For this review, use the dimensioned drawing (mm, ordinates from the lowest corner) and the shaded views. Coordinates: 2 decimals unless noted, no trailing zeros. Loops run counter-clockwise (first coordinate to the right, second up) from the corner with the lowest first, then second, coordinate; pieces in that order, holes last. Notation, with made-up numbers: (0, 32) - (45, 32) arc R18 cw to (45, 37) - close; hole circle Ø10 at (-1.5, -34). An arc over 180 degrees is marked (long way). Answer in a Markdown table with one row per item. Add a question column.
(1) We need section C-C, the plane z = 1.35. Write out the cut boundary in (x, y) (3 decimals).
(2) Clearance check with a flat-ended pin moving along its axis: pin 1 (6.5 mm diameter, centred on x = 10, y = 20, fed in from +Z). State where the tip first meets the part, or that it passes through.
(3) We need section D-D, the plane y = 55. Write out the cut boundary in (x, z).
(4) To check wall thickness, follow L1, parallel to Y at x = 9.5, z = 1.55; L2, parallel to Y at x = 12.5, z = 1.35; L3, parallel to X at y = 89.5, z = 0.85. State the ranges of each line that lie inside material, in increasing order. Write a range as [from, to].
(5) We need section A-A, the plane y = 89.5. Write out the cut boundary in (x, z).
(6) We need section B-B, the plane x = 10. Write out the cut boundary in (y, z).
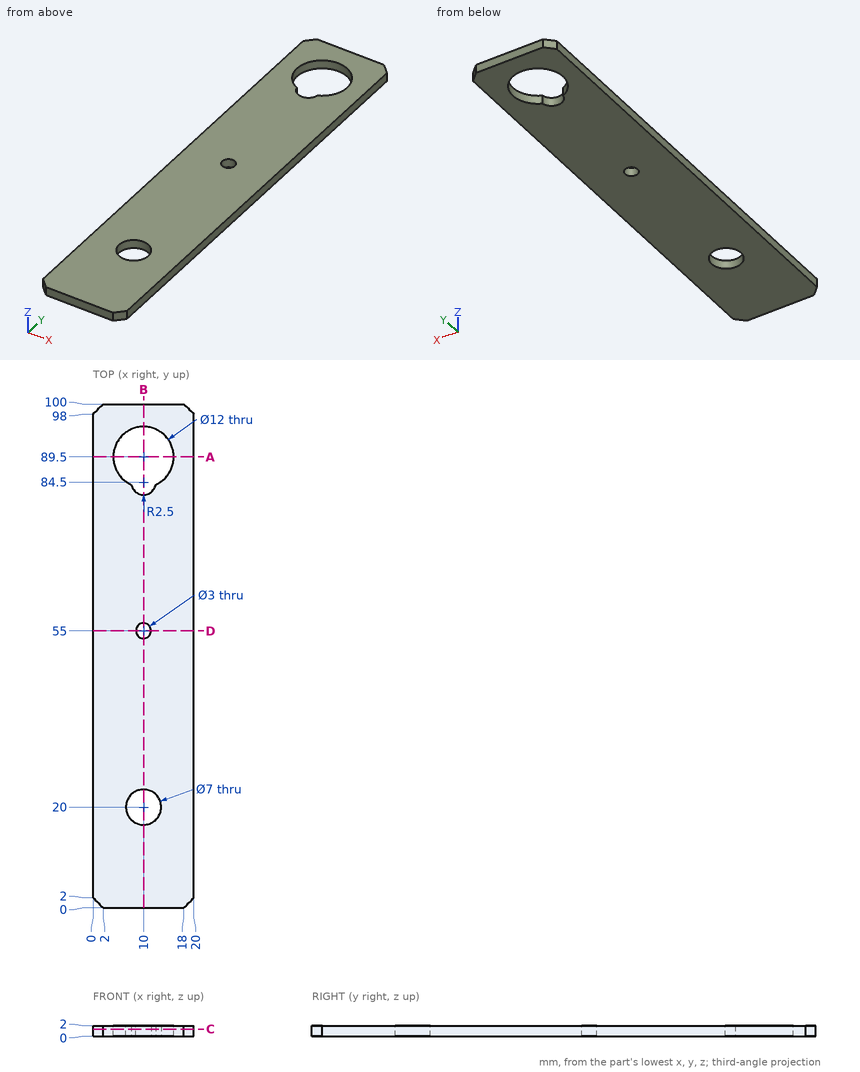
Responses:
| question | item | result |
|---|---|---|
| 1 | outline | (0, 2) - (2, 0) - (18, 0) - (20, 2) - (20, 98) - (18, 100) - (2, 100) - (0, 98) - close; hole circle Ø7 at (10, 20); hole (7.546, 84.025) arc R2.5 ccw to (12.454, 84.025) arc R6 ccw (long way) to start; hole circle Ø3 at (10, 55) |
| 2 | pin 1 | passes through |
| 3 | outline | (0, 0) - (8.5, 0) - (8.5, 2) - (0, 2) - close; (11.5, 0) - (20, 0) - (20, 2) - (11.5, 2) - close |
| 4 | L1 | y = [0, 16.54], [23.46, 53.59], [56.41, 82.05], [95.48, 100] |
| 4 | L2 | y = [0, 17.55], [22.45, 84.05], [94.95, 100] |
| 4 | L3 | x = [0, 4], [16, 20] |
| 5 | outline | (0, 0) - (4, 0) - (4, 2) - (0, 2) - close; (16, 0) - (20, 0) - (20, 2) - (16, 2) - close |
| 6 | outline | (0, 0) - (16.5, 0) - (16.5, 2) - (0, 2) - close; (23.5, 0) - (53.5, 0) - (53.5, 2) - (23.5, 2) - close; (56.5, 0) - (82, 0) - (82, 2) - (56.5, 2) - close; (95.5, 0) - (100, 0) - (100, 2) - (95.5, 2) - close |
